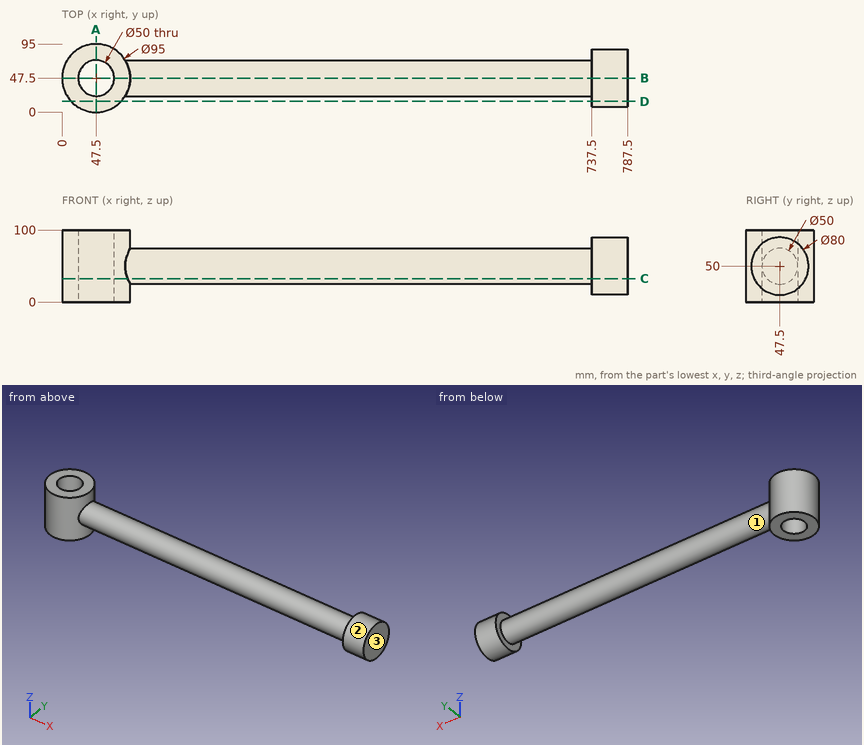
Could you check a few things on this drawing? It's one solid part, dimensions in mm from its lowest x, y, z. A direction names the side the tool comes from. Round coordinates to 2 decimals unless told otherwise and drop trailing zeros. Loops run counter-clockwise (first coordinate to the right, second up) from the corner with the lowest first, then second, coordinate; pieces in that order, holes last. Notation, with made-up numbers: (47, -37) -> (91, -37) arc R19 cw to (91, -18) -> close; hole circle Ø11 at (57.25, 72). An arc over 180 degrees is marked (long way). Write each question's results on one line, items separated by ' | '.
(1) If we section it at D-D, the plane y = 15: List the corners of the cut face in (x, z) for me, then the cut area to 3 significant figures.
Worked answers:
outline: (12.86, 0) -> (82.14, 0) -> (82.14, 100) -> (12.86, 100) -> close; (737.5, 26.68) -> (787.5, 26.68) -> (787.5, 73.32) -> (737.5, 73.32) -> close | area: 9,260 mm2
(2) If I drill on L1, parallel to X at y = 47, z = 76 (3 decimals); L2, parallel to X at y = 47, z = 52 (3 decimals); L3, parallel to Y at x = 47.5, z = 33.5, over which ranges is the centre line in solid material (lowest first)?
Worked answers:
L1: 0.003 to 22.505, 72.495 to 94.997, 737.5 to 787.5 | L2: 0.003 to 22.505, 72.495 to 787.5 | L3: 0 to 22.5, 72.5 to 95
(3) For P1, Ø6, axis at x = 91, z = 44.5, coming from the +Y side; P2, Ø2, axis at x = 685, z = 28, coming from the +Y side; P3, Ø1.5, axis at x = 377.5, y = 35, coming from the -Z side, each with a flat end and sliding along its axis, tell me the tip position at first contact or that it passes through.
Worked answers:
P1: y = 72.37 | P2: y = 61.06 | P3: z = 27.93
(4) For the marked faces 1, 2 and 3, which set-ups out of +Z, -Z, +X, -X, +Y, -Y let a thin tool reach every point of the face, with its end or its side?
Worked answers:
face 1: none | face 2: +X | face 3: +Z, -Z, +X, +Y, -Y
(5) If we section it at B-B, the plane y = 47.5: List the corners of the cut face in (x, z) for me.
Worked answers:
outline: (0, 0) -> (22.5, 0) -> (22.5, 100) -> (0, 100) -> close; (72.5, 0) -> (95, 0) -> (95, 25) -> (737.5, 25) -> (737.5, 10) -> (787.5, 10) -> (787.5, 90) -> (737.5, 90) -> (737.5, 75) -> (95, 75) -> (95, 100) -> (72.5, 100) -> close
(6) If we section it at C-C, the plane z = 32.5: List the corners of the cut face in (x, y) for me.
Worked answers:
outline: (91.52, 29.65) -> (737.5, 29.65) -> (737.5, 11.53) -> (787.5, 11.53) -> (787.5, 83.47) -> (737.5, 83.47) -> (737.5, 65.35) -> (91.52, 65.35) arc R47.5 ccw (long way) to start; hole circle Ø50 at (47.5, 47.5)
(7) If we section it at A-A, the plane x = 47.5: List the corners of the cut face in (y, z) for me, then the cut area to 3 significant figures.
Worked answers:
outline: (0, 0) -> (22.5, 0) -> (22.5, 100) -> (0, 100) -> close; (72.5, 0) -> (95, 0) -> (95, 100) -> (72.5, 100) -> close | area: 4,500 mm2
